Here's how the part is built. I have some questions about the finished solid (model axes, mm). Round coordinates to 2 decimals unless told otherwise and drop trailing zeros. Put each result on its own line as item: value. Start each with the question number.
1. Suppose I cut it at A-A (x = -11.5). Count the separate pieces of the cut face and the enclosed holes in it, then the cut area to 3 significant figures.
2. I need wall thicknesses on probe 1 along Z at (x, y) = (-25, -48); probe 2 along Z at (x, y) = (13.5, -49.2); probe 3 along Y at (x, z) = (13.5, 83.5). Which ranges of each line are inside material? Lowest first, please. Write a range as from..to.
3. For pin 1 (4 mm diameter, centred on x = -13.5, y = -140.5, fed in from +Z); pin 2 (3 mm diameter, centred on x = 13, z = 2.5, fed in from +Y); pin 3 (4 mm diameter, centred on x = -16.5, z = 17.5, fed in from +Y); pin 4 (3 mm diameter, centred on x = -0.5, y = -103, fed in from +Z), each with a flat end and sliding along its axis, tell me the tip position at first contact or that it passes through.
Autodesk Inventor part; units mm, degrees
ref_plane "Plano de trabajo3" through (29.25, 58.5, 1) normal (0, 0, 1) x (1, 0, 0)
ref_plane "Plano de trabajo4" through (-5.75, -5, -2.5) normal (1, 0, 0) x (0, 0, -1)
ref_plane "Plano de trabajo5" through (-27.5, -47.4, 0) normal (0, -1, 0) x (1, 0, 0)
sketch "Boceto1" plane through (0, 0, 0) normal (0, 0, 1) x (1, 0, 0)
  line L0 (81, 20) -> (81, 63.5)
  line L1 (-27.5, 63.5) -> (-27.5, -5)
  line L2 (-27.5, -5) -> (16, -5)
  line L3 (16, -5) -> (16, 20)
  line L4 (11, 25) -> (11, -5)
  line L5 (-22.5, 58.5) -> (-22.5, -5)
  line L6 (11, 25) -> (81, 25)
  line L7 (-27.5, 63.5) -> (81, 63.5)
  line L8 (-22.5, 58.5) -> (81, 58.5)
  line L9 (16, 20) -> (81, 20)
  point P0 (0, 0)
  dimension "d7" = 5
  dimension "d68" = 5
  dimension "d69" = 33.5
  dimension "d74" = 5
  dimension "d75" = 33.5
  dimension "d76" = 5
  dimension "d77" = 70
  dimension "d111" = 30
extrude "Extrusión1" add sketch "Boceto1" against normal blind 2.5
extrude "Extrusión2" add sketch "Boceto1" along normal blind 1 contours L9 L3 L2 L4 L6 L0 | L8 L5 L2 L1 L7 L0
ref_plane "Plano de trabajo3" through (29.25, 58.5, 1) normal (0, 0, 1) x (1, 0, 0)
mirror "Simetría3" about plane through (29.25, 58.5, 1) normal (0, 0, 1) of "Extrusión2", "Extrusión1"
sketch "Boceto6" plane through (-27.5, 63.5, 4.5) normal (0, 0, 1) x (1, 0, 0)
  line L0 (108.5, -43.5) -> (43.5, -43.5)
  line L1 (0, -68.5) -> (0, 0)
  line L2 (0, -43.5) -> (0, -51.5)
  line L3 (43.5, -43.5) -> (43.5, -68.5)
  line L4 (0, -43.5) -> (38.5, -43.5)
  line L5 (38.5, -68.5) -> (38.5, -38.5)
  line L6 (0, -51.5) -> (38.5, -51.5)
  line L7 (38.5, -43.5) -> (38.5, -51.5)
  point P0 (27.5, -63.5)
  point P1 (43.5, -51.5)
  dimension "d78" = 8
extrude "Extrusión11" cut sketch "Boceto6" against normal blind 4.5
sketch "Boceto7" plane through (-27.5, -5, -2.5) normal (-1, 0, 0) x (0, 0, 1)
  line L0 (0, 0) -> (0, 68.5)
  line L1 (0, 0) -> (0, -42.4)
  line L2 (0, 0) -> (7, 0)
  line L3 (0, 0) -> (7, 0)
  line L4 (7, 0) -> (7, -42.4)
  line L5 (0, -42.4) -> (86.5, -192.2224)
  line L6 (86.5, -192.2224) -> (89, -192.2224)
  line L7 (89, -192.2224) -> (92.375, -190.2738)
  line L8 (2.5, 0) -> (2.5, -42.4)
  line L9 (0, 0) -> (7, 0)
  line L10 (0, 0) -> (2.5, 0)
  line L11 (86.5, -192.2224) -> (89, -192.2224)
  line L12 (89, -192.2224) -> (92.375, -190.2738)
  line L13 (2.5, -42.4) -> (89, -192.2224)
  line L14 (0, -42.4) -> (-1.0904, -42.4)
  line L15 (7, -42.4) -> (92.375, -190.2738)
  line L16 (86.5, -187.8923) -> (89.875, -185.9437)
  point P0 (2.5, 5)
  point P1 (4.5, 0)
  point P2 (-0.5452, -42.4)
  dimension "d81" = 42.4
  dimension "d82" = 173
  dimension "d88" = 120
  dimension "d108" = 5
ref_plane "Plano de trabajo4" through (-5.75, -5, -2.5) normal (1, 0, 0) x (0, 0, -1)
extrude "Extrusión12" add sketch "Boceto7" against normal blind 21.75 contours L2 L8 L13 L6 L5 L1
extrude "Extrusión13" add sketch "Boceto7" against normal blind 5 contours L2 L4 L15 L16 L13 L8
extrude "Extrusión14" add sketch "Boceto7" against normal blind 21.75 contours L13 L16 L15 L7
mirror "Simetría4" about plane through (-5.75, -5, -2.5) normal (1, 0, 0) of "Extrusión12", "Extrusión13", "Extrusión14"
sketch "Boceto8" plane through (-22.5, -47.4, 0) normal (0, 0.5, 0.866) x (1, 0, 0)
  line L0 (0, 0) -> (33.5, 0)
  line L1 (16.75, 0) -> (16.75, -5)
  circle A0 centre (16.75, -15.25) radius 10.25
  line L2 (16.75, -25.5) -> (16.75, -30.5)
  circle A1 centre (16.75, -41.5) radius 11
  line L3 (16.75, -52.5) -> (16.75, -57.5)
  circle A2 centre (16.75, -68.69) radius 11.19
  line L4 (16.75, -79.88) -> (16.75, -84.88)
  circle A3 centre (16.75, -96.38) radius 11.5
  line L5 (16.75, -107.88) -> (16.75, -112.88)
  circle A4 centre (16.75, -125.07) radius 12.19
  line L6 (16.75, -137.26) -> (16.75, -142.26)
  circle A5 centre (16.75, -155.01) radius 12.75
  point P0 (22.5, 41.0496)
  dimension "d105" = 25.5
  dimension "d94" = 5
  dimension "d95" = 20.5
  dimension "d96" = 5
  dimension "d97" = 5
  dimension "d98" = 5
  dimension "d99" = 5
  dimension "d100" = 5
  dimension "d101" = 22
  dimension "d102" = 22.38
  dimension "d103" = 23
  dimension "d104" = 24.38
extrude "Extrusión15" cut sketch "Boceto8" against normal blind 21.75
sketch "Boceto9" plane through (-27.5, 63.5, -2.5) normal (-1, 0, 0) x (0, 0, 1)
  line L0 (2.5, -51.5) -> (2.5, -110.9)
  line L1 (0, 0) -> (0, -110.9)
  line L2 (0, -110.9) -> (2.5, -110.9)
  line L3 (2.5, -110.9) -> (2.5, -70.9)
  line L4 (2.5, -70.9) -> (0, -70.9)
  line L5 (0, -70.9) -> (0, -110.9)
  line L6 (0, -43.5) -> (0, -110.9)
  line L7 (0, -102.4) -> (2.5, -102.4)
  point P0 (2.5, -63.5)
  point P1 (7, -110.9)
  dimension "d109" = 2.5
  dimension "d110" = 40
  dimension "d112" = 31.5
extrude "Extrusión16" cut sketch "Boceto9" against normal through all contours L0 L7 L1 L4
ref_plane "Plano de trabajo5" through (-27.5, -47.4, 0) normal (0, -1, 0) x (1, 0, 0)
ref_plane "Plano de trabajo6" through (-27.5, -47.4, 0) normal (0, -1, 0) x (1, 0, 0)
sketch "Boceto11" plane through (-27.5, -47.4, 0) normal (0, -1, 0) x (1, 0, 0)
  line L0 (43.5, 4.5) -> (38.5, 4.5)
  line L1 (38.5, 0) -> (38.5, 4.5)
  line L2 (5, 0) -> (38.5, 0)
  line L3 (5, 4.5) -> (5, 0)
  line L4 (0, 4.5) -> (5, 4.5)
  line L5 (0, -2.5) -> (0, 4.5)
  line L6 (0, -2.5) -> (43.5, -2.5)
  line L7 (43.5, 4.5) -> (43.5, -2.5)
  line L8 (0, 0) -> (0, -2.5)
  line L9 (43.5, -2.5) -> (43.5, 4.5)
  circle A0 centre (2.5, 2) radius 1.25
  line L10 (108.5, 2) -> (5, 2)
  circle A1 centre (41, 2) radius 1.25
  circle A2 centre (11.5, -1.25) radius 0.75
  circle A3 centre (21.5, -1.25) radius 0.75
  circle A4 centre (31.5, -1.25) radius 0.75
  point P0 (27.5, 0)
  dimension "d117" = 2.5
  dimension "d118" = 2.5
  dimension "d119" = 38.5
  dimension "d120" = 1.5
  dimension "d121" = 1.5
  dimension "d122" = 1.5
  dimension "d123" = 10
  dimension "d124" = 10
extrude "Extrusión18" add sketch "Boceto11" along normal blind 2.5 contours A1 L10 | L10 A1 | A0
extrude "Extrusión19" cut sketch "Boceto11" against normal blind 2.5 contours A2 | A3 | A4
sketch "Boceto12" plane through (-27.5, -47.4, 0) normal (0, -1, 0) x (1, 0, 0)
  line L0 (0, -2.5) -> (0, 84)
  line L1 (0, 4.5) -> (108.5, 4.5)
  line L2 (0, -2.5) -> (108.5, -2.5)
  line L3 (108.5, -2.5) -> (108.5, 4.5)
  line L4 (108.5, 4.5) -> (0, 4.5)
  line L5 (0, 4.5) -> (0, -2.5)
  point P0 (27.5, 0)
extrude "Extrusión20" cut sketch "Boceto12" against normal through all
extrude "Extrusión21" add sketch "Boceto11" against normal blind 2.4 contours A2 | A3 | A4
extrude "Extrusión22" cut sketch "Boceto11" along normal blind 2.6 contours A1 L10 | L10 A1 | A0
equation "\"d105\" = UnSol"
equation "\"d94\" = razon"
equation "\"d95\" = diezcen"
equation "\"d96\" = razon"
equation "\"d97\" = razon"
equation "\"d98\" = razon"
equation "\"d99\" = razon"
equation "\"d100\" = razon"
equation "\"d101\" = cincuentacen"
equation "\"d102\" = dossol"
equation "\"d103\" = veintecen"
equation "\"d104\" = cincosol"
equation "\"UnSol\" = 25.5"
equation "\"diezcen\" = 20.5"
equation "\"veintecen\" = 23"
equation "\"cincuentacen\" = 22"
equation "\"dossol\" = 22.38"
equation "\"cincosol\" = 24.38"
equation "\"razon\" = 5"
properties part number "V2"
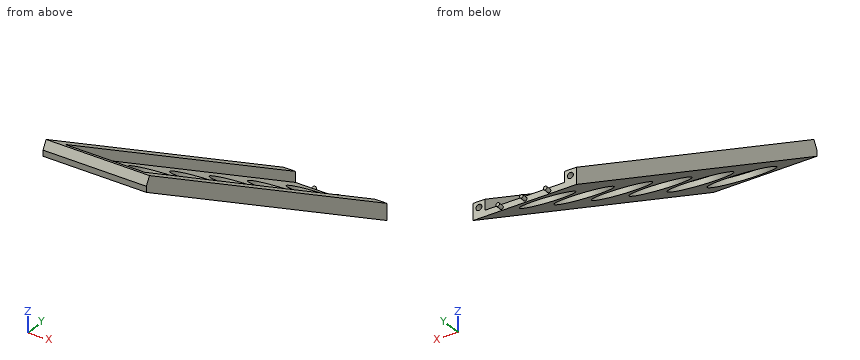
Verdict:
1. separate pieces: 7
1. enclosed holes: 0
1. area: 136 mm^2
2. probe 1: z = -2.15..0.75, 3.25..4.85
2. probe 2: z = -1.46..0.75, 3.25..5.54
2. probe 3: y = -196.36..-184.23
3. pin 1: stops at z = 54.91
3. pin 2: stops at y = -47.4
3. pin 3: stops at y = -74.25
3. pin 4: passes through
